The drawing under review shows one solid part. Ordinate dimensions are in mm from its lowest x, y, z. A direction names the side the tool comes from. Coordinates: 2 decimals unless noted, no trailing zeros. Write each loop counter-clockwise with the first axis right and the second up, starting at its lowest first coordinate (ties: lowest second). Pieces come first, ordered by that corner, then holes. Notation, with made-up numbers: M -18,6 L -6,6 A31 ccw -6,35 Z; hole C -13,-32 d2. An arc over 180 degrees is marked long. Write item = value, one per line.
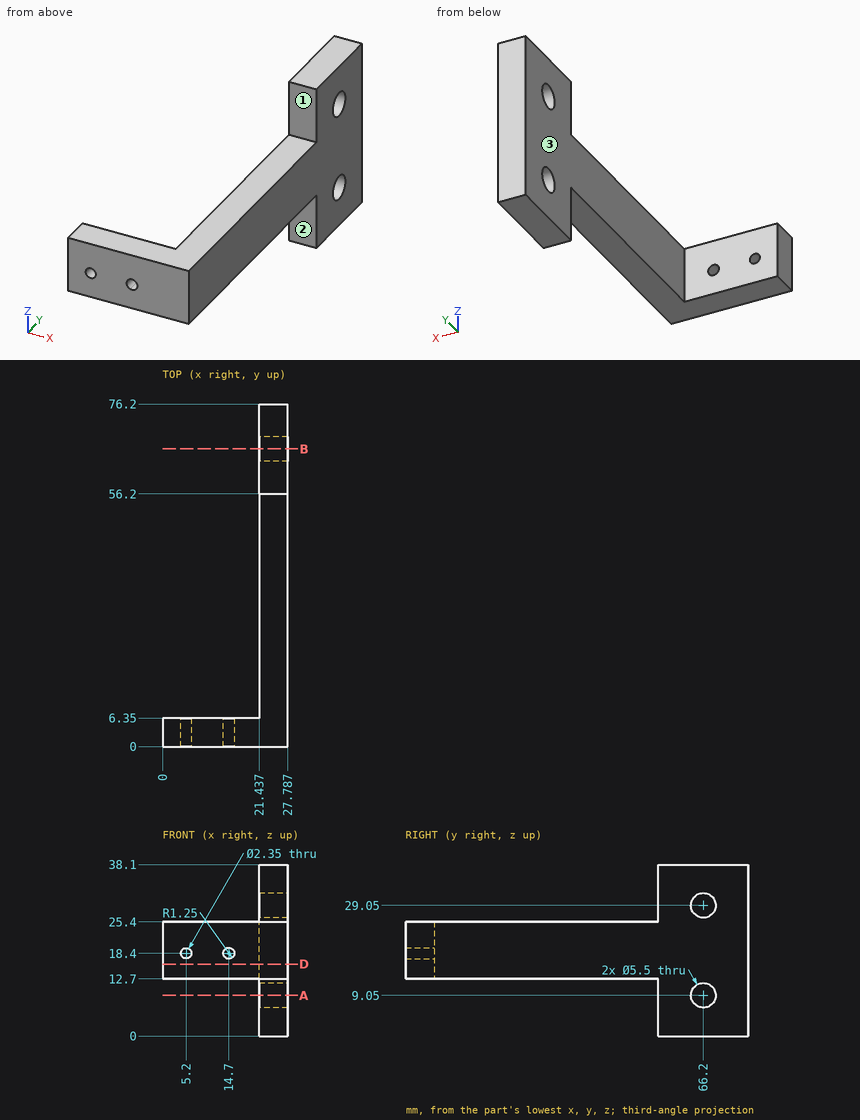
Q1. For P1, Ø4.5, axis at y = 66.2, z = 9.05, coming from the +X side; P2, Ø6.5, axis at x = 10.5, z = 19.5, coming from the +Y side; P3, Ø12, axis at y = 61, z = 18, coming from the -X side; P4, Ø1.9, axis at x = 23, z = 3, coming from the -Y side, all flat-tipped, find the tip position at first contact; note any pin that passes through.
Check result:
P1 = through
P2 = 6.35
P3 = 21.44
P4 = 56.2
Q2. Consider section A-A, the plane z = 9.05. State the section outline as (x, y) points.
Check result:
outline = M 21.44,56.2 L 27.79,56.2 L 27.79,63.45 L 21.44,63.45 Z; M 21.44,68.95 L 27.79,68.95 L 27.79,76.2 L 21.44,76.2 Z
Q3. Wall thickness on line 1 (Z direction, x = 22, y = 66); line 2 (Y direction, x = 15.5, z = 20); line 3 (Y direction, x = 22.5, z = 29.05): over which ranges is each line inside the solid? List them lowest first.
Check result:
line_1 = 0 to 6.31, 11.79 to 26.31, 31.79 to 38.1
line_2 = 0 to 6.35
line_3 = 56.2 to 63.45, 68.95 to 76.2
Q4. Consider section D-D, the plane z = 16. State the section outline as (x, y) points, and give its area (3 significant figures).
Check result:
outline = M 0,0 L 27.79,0 L 27.79,76.2 L 21.44,76.2 L 21.44,6.35 L 0,6.35 Z
area = 620 mm²
Q5. Machinability: for the marked faces 1, 2 and 3, which of the approach directions +Z, -Z, +X, -X, +Y, -Y give a long, thin tool a straight path to every point of the face, cutting with its end or side? Answer none if there is none.
Check result:
face_1 = +Z, +X, -X, -Y
face_2 = -Z, +X, -X, -Y
face_3 = +Z, -Z, -X, +Y
Q6. Consider section B-B, the plane y = 66.2. State the section outline as (x, z) points, and give its area (3 significant figures).
Check result:
outline = M 21.44,0 L 27.79,0 L 27.79,6.3 L 21.44,6.3 Z; M 21.44,11.8 L 27.79,11.8 L 27.79,26.3 L 21.44,26.3 Z; M 21.44,31.8 L 27.79,31.8 L 27.79,38.1 L 21.44,38.1 Z
area = 172 mm²
